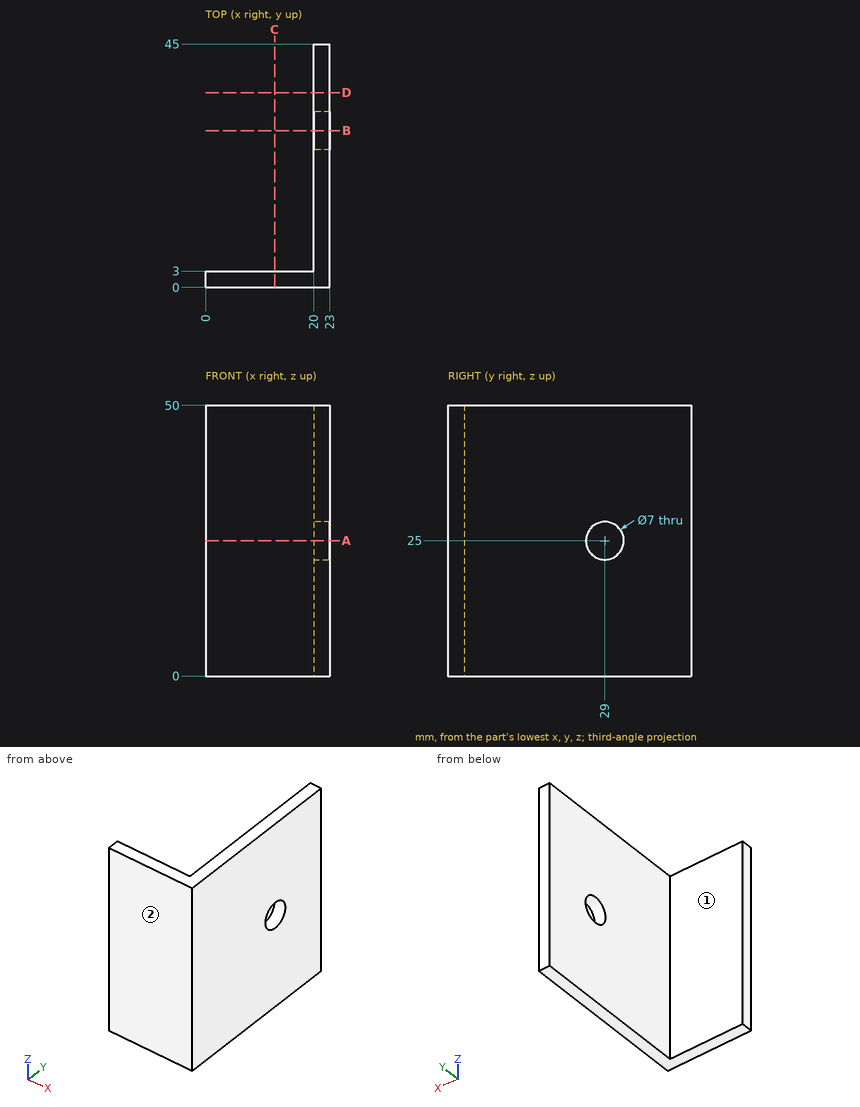
Job drawing, mm, ordinate dimensions from the low corner. One solid piece. A direction names the side the tool comes from. Coordinates: 2 decimals unless noted, no trailing zeros. Order: outer loops, then holes, each group sorted by start corner. A loop starts at its lowest first (then second) coordinate and runs counter-clockwise, first axis right, second up. Notation, with made-up numbers: (80.5, 2) -> (106.5, 2) arc R22 cw to (106.5, 19) -> close; hole circle Ø8 at (76.5, -36). An arc over 180 degrees is marked (long way). Return JSON: item names as keys, results as strings. Group by question number.
Item 1: Saw through at A-A on z = 25. Write the cut outline in (x, y), then the cut area to 3 significant figures.
Item 2: Saw through at C-C on x = 12.75. Write the cut outline in (y, z).
Item 3: Tool access for the marked faces 1 and 2: list every direction of +Z, -Z, +X, -X, +Y, -Y with a clear straight run to the whole face (end or side of a thin tool).
Item 4: Flat gauge pin, fed straight in: P1, Ø3, axis at y = 34.5, z = 44.5, coming from the -X side. Where does the tip first touch, or does it go through?
Item 5: Saw through at D-D on y = 36. Write the cut outline in (x, z).
Item 6: Saw through at B-B on y = 29. Write the cut outline in (x, z), then the cut area to 3 significant figures.
Item 7: Wall check: line 1 along Y through (x, z) = (21.6, 25); line 2 along Y through (x, z) = (6.5, 17.5); line 3 along X through (y, z) = (12, 36). Give the ranges that are in metal, low to high. Write a range as [from, to].
Values found:
{
 "1": {"outline": "(0, 0) -> (23, 0) -> (23, 25.5) -> (20, 25.5) -> (20, 3) -> (0, 3) -> close; (20, 32.5) -> (23, 32.5) -> (23, 45) -> (20, 45) -> close", "area": "174 mm2"},
 "2": {"outline": "(0, 0) -> (3, 0) -> (3, 50) -> (0, 50) -> close"},
 "3": {"face 1": "+Z, -Z, -X, +Y", "face 2": "+Z, -Z, +X, -X, -Y"},
 "4": {"P1": "stops at x = 20"},
 "5": {"outline": "(20, 0) -> (23, 0) -> (23, 50) -> (20, 50) -> close"},
 "6": {"outline": "(20, 0) -> (23, 0) -> (23, 21.5) -> (20, 21.5) -> close; (20, 28.5) -> (23, 28.5) -> (23, 50) -> (20, 50) -> close", "area": "129 mm2"},
 "7": {"line 1": "y = [0, 25.5], [32.5, 45]", "line 2": "y = [0, 3]", "line 3": "x = [20, 23]"}
}
